Could you check a few things on this model? Use its own coordinates, in mm. Face numbers are marked on the shaded views. A direction names the side the tool comes from. Coordinates: 2 decimals unless noted, no trailing zeros. Loops run counter-clockwise (first coordinate to the right, second up) from the corner with the lowest first, then second, coordinate; pieces in that order, holes last. Notation, with made-up numbers: (18, 16.5) - (76, 16.5) arc R14 cw to (76, 24.5) - close; hole circle Ø11 at (32.25, -0.75). An arc over 180 degrees is marked (long way). Put each result on its own line as item: value. Start each with the question number.
```python
from build123d import *

# Parameters (mm, degrees)
F2_R = 9.525
F4_R = 5.08


# Not quite as in the source:
# - a fillet or chamfer that OpenCascade refuses, or shapes differently, is made with other operations: its cross-section is extruded or revolved along the edge and cut away or added


with BuildPart() as f1:
    # F0 (on Front) → F1 (revolve)
    with BuildSketch(Plane.XZ):
        Polygon((0, 4.7625), (0, 0), (64.516, 0), (64.516, 9.525), (8.89, 9.525), (8.89, 4.7625), align=None)
    revolve(axis=Axis((32.258, 0, 0), (1, 0, 0)))

    # F2
    f2_edges = [f1.edges().sort_by_distance(p)[0] for p in [
        (64.516, 0, -9.525),
    ]]
    fillet(f2_edges, radius=F2_R)

    # F3: fillet of radius 5.08 on 1 edges, made by hand

    # F3_s1 → F3_t2 (revolve)
    with BuildSketch(Plane.XZ):
        with BuildLine():
            ThreePointArc((8.89, 9.525), (7.2979698235, 6.1398455468), (3.8199315833, 4.7625))
            Line((3.8199315833, 4.7625), (8.89, 4.7625))
            Line((8.89, 4.7625), (8.89, 9.525))
        make_face()
    revolve(axis=Axis((8.89, 0, 0), (1, 0, 0)))

    # F4
    f4_edges = [f1.edges().sort_by_distance(p)[0] for p in [
        (8.89, 0, -9.525),
    ]]
    fillet(f4_edges, radius=F4_R)


solid = f1.part
```
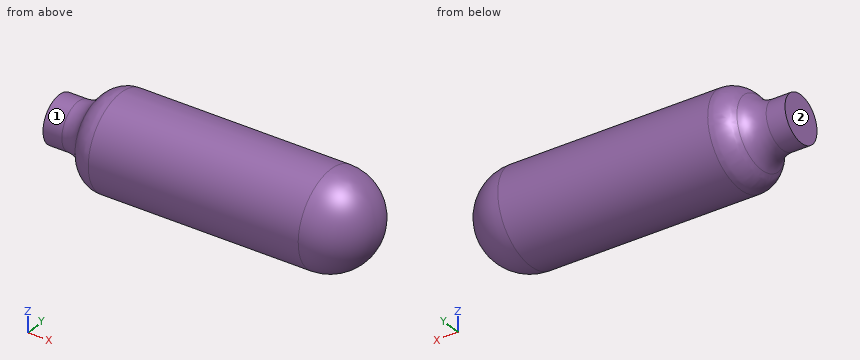
(1) For pin 1 Ø2 at (x, y) = (53, -7) entering from -Z; pin 2 Ø4 at (x, z) = (24.5, 6) entering from +Y; pin 3 Ø10 at (y, z) = (5.5, -0.5) entering from +X, each with a flat end and sliding along its axis, tell me the tip position at first contact or that it passes through.
(2) I want a section at A-A on x = 44. List the corners of the cut face in (y, z) for me (3 decimals), and give its area (3 significant figures).
(3) Which directions (+Z, -Z, +X, -X, +Y, -Y) give clear straight access to the entire face, cutting with the end or side of a thin tool? Please do the marked faces 1 and 2.
(4) I need wall thicknesses on L1, parallel to Z at x = 54.5, y = -0.25; L2, parallel to Z at x = 22.5, y = -3; L3, parallel to X at y = 4, z = -0.5. Which ranges of each line are inside material? Lowest first, please. Write a range as [from, to].
Answer sheet:
1. pin 1: stops at z = -7.4
1. pin 2: stops at y = 8.64
1. pin 3: stops at x = 64.5
2. outline: circle Ø19.05 at (0, 0)
2. area: 285 mm^2
3. face 1: -X
3. face 2: +Z, -Z, -X, +Y, -Y
4. L1: z = [-9.52, 9.52]
4. L2: z = [-9.04, 9.04]
4. L3: x = [0, 63.62]
